The model under review builds one solid part; all positions refer to its coordinate system, in mm. A direction names the side the tool comes from. Coordinates: 2 decimals unless noted, no trailing zeros. Order: outer loops, then holes, each group sorted by start corner. A loop starts at its lowest first (then second) coordinate and runs counter-clockwise, first axis right, second up. Notation, with made-up numbers: (-29.5, 73) -> (13.5, 73) arc R27 cw to (13.5, 105) -> close; hole circle Ø8 at (50.5, -13). An arc over 180 degrees is marked (long way). Use one line per item in the form item = value. Start each with the question number.
(1) Take a section at B-B (y = 12). State the section outline as (x, z) points.
(2) Mouldability with a two-part tool opening along X and no side actions: class faces 1 (the cylindrical face through (-100.935, -23.739, 2.535)), 2 (the flat face through (-3, 1, 0)) as +X half, -X half, draft (parallel to the pull), parting line (faces both ways), or undercut.
(3) Take a section at C-C (x = -66.5). State the section outline as (y, z) points.
(4) Take a section at A-A (x = 229). State the section outline as (y, z) points (3 decimals).
(5) For faces 3 (the cylindrical face through (65.78, -25.565, 0.477)), 4 (the cylindrical face through (-100.935, 21.261, 2.535)), 5 (the cylindrical face through (198.22, 29.912, 4.363)), list the 3-axis set-ups (+Z, -Z, +X, -X, +Y, -Y) from which the entire face can be reached by the end or side of a thin tool; tool diameter is ignored.
(6) Wall thickness on line 1 along Y through (x, z) = (35, 2.95) (3 decimals); line 2 along X through (y, z) = (17.5, 1.7); line 3 along Y through (x, z) = (-199, 3.15): over which ranges is each line inside the solid? List them lowest first.
(7) Take a section at D-D (z = 1.1). State how many separate pieces and enclosed holes the cut face has, then the cut area to 3 significant figures.
(8) Insertion check: pin 1 Ø5 at (x, y) = (126, 24) entering from -Z. The pin has a flat end and moves straight along its axis. Give the tip position at first contact, or say it passes through.
```python
from build123d import *

# Parameters (mm, degrees)
F0_W     = 478
F0_H     = 85
F1_DEPTH = 5
F2_D     = 8.25
F5_DEPTH = 54.637947


with BuildPart() as f1:
    # F0 (on Top) → F1 (new body)
    with BuildSketch(Plane.XY):
        Rectangle(F0_W, F0_H)
    extrude(amount=F1_DEPTH)

    # F2 (through all)
    with Locations(Plane(origin=(0, 0, 0), x_dir=(1, 0, 0), z_dir=(0, 0, -1))):
        with Locations((-229, 22.5), (-229, -22.5), (-167, 22.5), (-167, -22.5), (-97, 22.5), (-97, -22.5), (-35, 22.5), (-35, -22.5), (35, 22.5), (35, -22.5), (97, 22.5), (97, -22.5), (167, 22.5), (167, -22.5), (229, 22.5), (229, -22.5)):
            Hole(F2_D / 2)

    # F4 (on face) → F5 (cut, through all)
    with BuildSketch(Plane(origin=(0, 15.097957, -17.993044), x_dir=(1, 0, 0), z_dir=(0, -0.642788, 0.766044))):
        with BuildLine():
            ThreePointArc((188, -9.279173), (198, -19.279173), (208, -9.279173))
            Line((208, -9.279173), (208, 15.720827))
            ThreePointArc((208, 15.720827), (198, 25.720827), (188, 15.720827))
            Line((188, 15.720827), (188, -9.279173))
        make_face()
        with BuildLine():
            Line((56, 15.720827), (56, -9.279173))
            ThreePointArc((56, -9.279173), (66, -19.279173), (76, -9.279173))
            Line((76, -9.279173), (76, 15.720827))
            ThreePointArc((76, 15.720827), (66, 25.720827), (56, 15.720827))
        make_face()
        with BuildLine():
            Line((-76, 15.720827), (-76, -9.279173))
            ThreePointArc((-76, -9.279173), (-66, -19.279173), (-56, -9.279173))
            Line((-56, -9.279173), (-56, 15.720827))
            ThreePointArc((-56, 15.720827), (-66, 25.720827), (-76, 15.720827))
        make_face()
        with BuildLine():
            Line((-208, 15.720827), (-208, -9.279173))
            ThreePointArc((-208, -9.279173), (-198, -19.279173), (-188, -9.279173))
            Line((-188, -9.279173), (-188, 15.720827))
            ThreePointArc((-188, 15.720827), (-198, 25.720827), (-208, 15.720827))
        make_face()
    extrude(amount=F5_DEPTH, mode=Mode.SUBTRACT)


solid = f1.part
```
Findings:
q1.outline = (-239, 0) -> (-208, 0) -> (-208, 5) -> (-239, 5) -> close; (-188, 0) -> (-76, 0) -> (-76, 5) -> (-188, 5) -> close; (-56, 0) -> (56, 0) -> (56, 5) -> (-56, 5) -> close; (76, 0) -> (188, 0) -> (188, 5) -> (76, 5) -> close; (208, 0) -> (239, 0) -> (239, 5) -> (208, 5) -> close
q2.face_1 = undercut
q2.face_2 = draft
q3.outline = (-42.5, 0) -> (-25.15, 0) -> (-29.35, 5) -> (-42.5, 5) -> close; (29.36, 5) -> (33.56, 0) -> (42.5, 0) -> (42.5, 5) -> close
q4.outline = (-42.5, 0) -> (-26.625, 0) -> (-26.625, 5) -> (-42.5, 5) -> close; (-18.375, 0) -> (18.375, 0) -> (18.375, 5) -> (-18.375, 5) -> close; (26.625, 0) -> (42.5, 0) -> (42.5, 5) -> (26.625, 5) -> close
q5.face_3 = +Z
q5.face_4 = +Z, -Z
q5.face_5 = -Z
q6.line_1 = -42.5 to -26.625, -18.375 to 18.375, 26.625 to 42.5
q6.line_2 = -239 to -208, -188 to -76, -56 to 56, 76 to 188, 208 to 239
q6.line_3 = -42.5 to -27.74, 30.87 to 42.5
q7.separate_pieces = 1
q7.enclosed_holes = 20
q7.area = 35,500 mm²
q8.pin_1 = 0
